Design review of the part built by this model. Coordinates are the model's own, in mm. A direction names the side the tool comes from. Round coordinates to 2 decimals unless told otherwise and drop trailing zeros. Write each loop counter-clockwise with the first axis right and the second up, starting at its lowest first coordinate (ties: lowest second). Pieces come first, ordered by that corner, then holes. Notation, with made-up numbers: M 78,1.25 L 92,1.25 A19 ccw 92,30.25 Z; hole C 36.25,28 d1. An arc over 180 degrees is marked long. Use CSV: the item, a comma, the result in double quotes.
from build123d import *

# Parameters (mm, degrees)
SKETCH001_W  = 40.8
SKETCH001_H  = 30.6
PAD001_DEPTH = 1
SKETCH_W     = 47.8
SKETCH_H     = 34.6
PAD_DEPTH    = 0.95
PAD002_DEPTH = 5.65
PAD003_DEPTH = 0.13


with BuildPart() as part:
    # Sketch001 → Pad001 (new body)
    with BuildSketch(Plane.XY):
        Rectangle(SKETCH001_W, SKETCH001_H)
    extrude(amount=PAD001_DEPTH)

    # Sketch → Pad (join, symmetric)
    with BuildSketch(Plane.XY):
        with Locations((1.5, 0)):
            Rectangle(SKETCH_W, SKETCH_H)
    extrude(amount=PAD_DEPTH, both=True)

    # Sketch002 → Pad002 (join, symmetric)
    with BuildSketch(Plane.XZ):
        with BuildLine():
            Line((25.4, 0.5), (25.62, 0.5))
            ThreePointArc((25.77, 0.35), (25.726066, 0.456066), (25.62, 0.5))
            Line((25.77, 0.35), (25.77, -7.27))
            ThreePointArc((25.62, -7.42), (25.726066, -7.376066), (25.77, -7.27))
            Line((25.4, -7.42), (25.62, -7.42))
            Line((25.4, -7.55), (25.4, -7.42))
            Line((25.65, -7.55), (25.4, -7.55))
            ThreePointArc((25.65, -7.55), (25.826777, -7.476777), (25.9, -7.3))
            Line((25.9, 0.38), (25.9, -7.3))
            ThreePointArc((25.9, 0.38), (25.826777, 0.556777), (25.65, 0.63))
            Line((25.4, 0.63), (25.65, 0.63))
            Line((25.4, 0.5), (25.4, 0.63))
        make_face()
    extrude(amount=PAD002_DEPTH, both=True)

    # Sketch003 (on DatumPlane) → Pad003 (join)
    with BuildSketch(Plane(origin=(0, 0, -7.55), x_dir=(-1, 0, 0), z_dir=(0, 0, -1))):
        Polygon((-25.4, -5.65), (-25.4, 5.65), (-23.393548, 5.65), (-20.2, 7.9), (-10.6, 7.9), (-10.6, -4.1), (-20.2, -4.1), (-22.4, -5.65), align=None)
    extrude(amount=-PAD003_DEPTH)


solid = part.part
1) For pin 1 Ø2.5 at (y, z) = (-0.5, -4.5) entering from -X; pin 2 Ø1.1 at (x, z) = (23.5, -5.5) entering from -Y; pin 3 Ø1.5 at (x, y) = (21, 11) entering from -Z; pin 4 Ø0.6 at (y, z) = (8.5, 0) entering from +X, all flat-tipped, find the tip position at first contact; note any pin that passes through.
Answers:
pin 1,"x = 25.77"
pin 2,"through"
pin 3,"z = -0.95"
pin 4,"x = 25.4"
2) Machinability: for faces 4 (the face through (6.7, 15.5, 0.95)), 5 (the face through (-22.4, 0, 0)), which of the approach directions +Z, -Z, +X, -X, +Y, -Y give a long, thin tool a straight path to every point of the face, cutting with its end or side? Answer none if there is none.
Answers:
face 4,"+Z"
face 5,"+Z, -Z, -X, +Y, -Y"
3) Add section B-B on y = -1.5. Write out the cut boundary in (x, z).
Answers:
outline,"M -22.4,-0.95 L 25.4,-0.95 L 25.4,0.5 L 25.62,0.5 A0.15 cw 25.77,0.35 L 25.77,-7.27 A0.15 cw 25.62,-7.42 L 10.6,-7.42 L 10.6,-7.55 L 25.65,-7.55 A0.25 ccw 25.9,-7.3 L 25.9,0.38 A0.25 ccw 25.65,0.63 L 25.4,0.63 L 25.4,0.95 L 20.4,0.95 L 20.4,1 L -20.4,1 L -20.4,0.95 L -22.4,0.95 Z"
4) Wall thickness on line 1 along Z through (x, y) = (-10, -13.5); line 2 along X through (y, z) = (13.5, -0.25): over which ranges is each line inside the solid? List them lowest first. Write a range as [from, to].
Answers:
line 1,"[-0.95, 1]"
line 2,"[-22.4, 25.4]"
5) Add section D-D on z = -3. Write out the cut boundary in (x, y), then the cut area to 3 significant figures.
Answers:
outline,"M 25.77,-5.65 L 25.9,-5.65 L 25.9,5.65 L 25.77,5.65 Z"
area,"1.47 mm²"
6) The part is to be moulded in two halves that separate along Z. For faces 1 (the face through (25.4, 0, 0)), 2 (the face through (1, 17.3, 0)), 3 (the face through (0, 0, 1)), say which applies: released by +Z, released by -Z, zero draft, split by the parting line, or undercut.
Answers:
face 1,"undercut"
face 2,"zero draft"
face 3,"released by +Z"
7) Add section C-C on x = -16. Write out the cut boundary in (y, z).
Answers:
outline,"M -17.3,-0.95 L 17.3,-0.95 L 17.3,0.95 L 15.3,0.95 L 15.3,1 L -15.3,1 L -15.3,0.95 L -17.3,0.95 Z"
8) Add section A-A on x = 17. Write out the cut boundary in (y, z).
Answers:
outline,"M -17.3,-0.95 L 17.3,-0.95 L 17.3,0.95 L 15.3,0.95 L 15.3,1 L -15.3,1 L -15.3,0.95 L -17.3,0.95 Z; M -4.1,-7.55 L 7.9,-7.55 L 7.9,-7.42 L -4.1,-7.42 Z"
